Autodesk Inventor part; units mm, degrees
ref_plane "YZ Plane" through (0, 0, 0) normal (1, 0, 0) x (0, 1, 0)
ref_plane "XZ Plane" through (0, 0, 0) normal (0, 1, 0) x (-1, 0, 0)
ref_plane "XY Plane" through (0, 0, 0) normal (0, 0, 1) x (1, 0, 0)
sketch "Sketch1" plane through (0, 0, 0) normal (0, 1, 0) x (-1, 0, 0)
  line L0 (-16.8496, 81.8638) -> (105.0704, 81.8638)
  line L1 (105.0704, 81.8638) -> (105.0704, -7.0362)
  line L2 (105.0704, -7.0362) -> (-16.8496, -7.0362)
  line L3 (-16.8496, -7.0362) -> (-16.8496, 81.8638)
  point P0 (0, 0)
  dimension "d0" = 121.92
  dimension "d1" = 88.9
extrude "Extrusion1" add sketch "Sketch1" along normal blind 3.429
sketch "Sketch2" plane through (0, 3.429, 0) normal (0, 1, 0) x (1, 0, 0)
  line L0 (-105.0704, -81.8638) -> (16.8496, -81.8638)
  line L1 (16.8496, 7.0362) -> (-105.0704, 7.0362)
  line L2 (-105.0704, 7.0362) -> (-105.0704, -81.8638)
  circle A0 centre (-98.7204, -2.6158) radius 1.5875
  circle A1 centre (-98.7204, -72.2118) radius 1.5875
  circle A2 centre (-4.7404, -2.6158) radius 1.5875
  circle A3 centre (-4.7404, -72.2118) radius 1.5875
  point P0 (0, 0)
  dimension "d4" = 121.92
  dimension "d5" = 88.9
  dimension "d6" = 6.35
  dimension "d8" = 6.35
  dimension "d12" = 3.175
  dimension "d13" = 3.175
  dimension "d15" = 3.175
  dimension "d18" = 93.98
  dimension "d20" = 69.596
  dimension "d21" = 9.652
  dimension "d22" = 9.652
  dimension "d23" = 3.175
  dimension "d64" = 9.652
  dimension "d65" = 9.652
extrude "Extrusion3" cut sketch "Sketch2" against normal through all
sketch "Sketch4" plane through (0, 3.429, 0) normal (0, 1, 0) x (1, 0, 0)
  circle A0 centre (-98.7204, -2.6158) radius 1.5875
  circle A1 centre (-98.7204, -72.2118) radius 1.5875
  line L0 (16.8496, 7.0362) -> (-105.0704, 7.0362)
  line L1 (-105.0704, 7.0362) -> (-105.0704, -81.8638)
  line L2 (-101.8954, -78.6888) -> (-47.0314, -78.6888)
  line L3 (-47.0314, -78.6888) -> (-47.0314, 3.8612)
  line L4 (-47.0314, 3.8612) -> (-101.8954, 3.8612)
  line L5 (-101.8954, 3.8612) -> (-101.8954, -78.6888)
  circle A2 centre (-98.7204, -2.6158) radius 3.175
  circle A3 centre (-98.7204, -72.2118) radius 3.175
  point P0 (0, 0)
  dimension "d26" = 54.864
  dimension "d27" = 82.55
  dimension "d28" = 3.175
  dimension "d29" = 3.175
  dimension "d38" = 3.175
extrude "Extrusion4" add sketch "Sketch4" along normal blind 2.54 contours L5 L4 L3 L2
sketch "Sketch5" plane through (0, 3.429, 0) normal (0, 1, 0) x (1, 0, 0)
  line L0 (-47.0314, 3.8612) -> (-47.0314, -78.6888)
  line L1 (-47.0314, -37.4138) -> (-47.0314, -31.0638)
  line L2 (-47.0314, -31.0638) -> (-47.0314, -43.7638)
  line L3 (-47.0314, -43.7638) -> (-41.9514, -43.7638)
  circle A0 centre (-41.9514, -43.7638) radius 5.08
  circle A1 centre (-41.9514, -31.0638) radius 5.08
  point P0 (0, 0)
  dimension "d35" = 6.35
  dimension "d36" = 12.7
  dimension "d37" = 5.08
extrude "Extrusion5" cut sketch "Sketch5" against normal through all
sketch "Sketch6" plane through (0, 3.429, 0) normal (0, 1, 0) x (1, 0, 0)
  line L0 (-47.0314, -31.0638) -> (-47.0314, -43.7638)
  line L1 (-105.0704, 7.0362) -> (-105.0704, -81.8638)
  line L2 (-47.0314, -37.4138) -> (-40.6814, -37.4138)
  line L3 (-40.6814, -37.4138) -> (-40.6814, -65.3538)
  line L4 (-40.6814, -65.3538) -> (-40.6814, 3.1754)
  line L5 (-40.6814, 3.1754) -> (12.6586, 3.1754)
  line L6 (12.6586, 3.1754) -> (12.6586, -65.3538)
  line L7 (12.6586, -65.3538) -> (-40.6814, -65.3538)
  line L8 (-40.6814, -65.3538) -> (-40.6814, -63.0678)
  line L9 (-40.6814, -63.0678) -> (12.6586, -63.0678)
  line L10 (-40.6814, -63.0678) -> (-33.0614, -63.0678)
  line L11 (-33.0614, -63.0678) -> (-5.1214, -63.0678)
  circle A0 centre (-33.0614, -63.0678) radius 3.175
  circle A1 centre (-5.1214, -63.0678) radius 3.175
  line L12 (-40.6814, 3.1754) -> (-38.3954, 3.1754)
  line L13 (-38.3954, 3.1754) -> (-38.3954, -65.3538)
  line L14 (-38.3954, 3.1754) -> (-38.3954, -10.6168)
  circle A2 centre (-38.3954, -10.6168) radius 3.175
  line L15 (10.3726, 3.1754) -> (10.3726, -11.7598)
  circle A3 centre (10.3726, -11.7598) radius 3.175
  point P0 (0, 0)
  dimension "d39" = 6.35
  dimension "d40" = 27.94
  dimension "d41" = 68.5292
  dimension "d42" = 53.34
  dimension "d43" = 2.286
  dimension "d44" = 7.62
  dimension "d45" = 27.94
  dimension "d46" = 6.35
  dimension "d47" = 6.35
  dimension "d48" = 2.286
  dimension "d49" = 13.7922
  dimension "d50" = 6.35
  dimension "d51" = 14.9352
  dimension "d52" = 2.286
  dimension "d53" = 6.35
extrude "Extrusion6" add sketch "Sketch6" along normal blind 3.81 contours A2 L4 | L4 A2 L13 | L13 A2 | A0 L9 | L9 A0 L7 | L7 A0 | A1 L9 | L9 A1 L7 | L7 A1 | A3 L6 | A3 L6
sketch "Sketch7" plane through (-38.3954, 7.239, 10.6168) normal (0, 1, 0) x (1, 0, 0)
  circle A0 centre (48.768, -1.143) radius 3.175
  circle A1 centre (33.274, -52.451) radius 3.175
  circle A2 centre (5.334, -52.451) radius 3.175
  circle A3 centre (48.768, -1.143) radius 1.27
  point P0 (38.3954, 10.6168)
  dimension "d56" = 2.54
extrude "Extrusion7" add sketch "Sketch7" along normal blind 2.54 contours A3
sketch "Sketch8" plane through (-38.3954, 7.239, 10.6168) normal (0, 1, 0) x (1, 0, 0)
  circle A0 centre (0, 0) radius 3.175
  circle A1 centre (5.334, -52.451) radius 3.175
  circle A2 centre (33.274, -52.451) radius 3.175
  circle A3 centre (0, 0) radius 1.0605
  circle A4 centre (5.334, -52.451) radius 1.0605
  circle A5 centre (33.274, -52.451) radius 1.0604
  point P0 (38.3954, 10.6168)
  dimension "d59" = 2.1209
  dimension "d60" = 2.1209
  dimension "d61" = 2.1209
extrude "Extrusion8" cut sketch "Sketch8" against normal through all contours A3 | A4 | A5
properties part number "base_plate_r2"
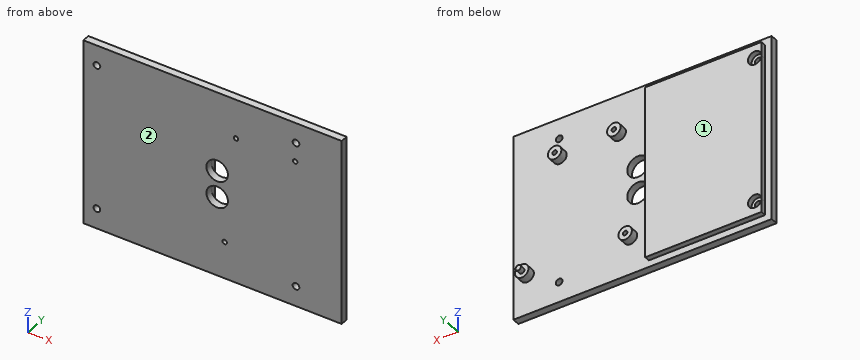
Design review of the part built by this model. Coordinates are the model's own, in mm. Face numbers are marked on the shaded views. A direction names the side the tool comes from. Round coordinates to 2 decimals unless told otherwise and drop trailing zeros. Write each loop counter-clockwise with the first axis right and the second up, starting at its lowest first coordinate (ties: lowest second). Pieces come first, ordered by that corner, then holes. Notation, with made-up numbers: (68, 31) -> (95, 31) arc R15 cw to (95, 54) -> close; hole circle Ø6 at (18, -13.5). An arc over 180 degrees is marked (long way). One line per item, written item: value. Start each with the question number.
Q1. Add section B-B (x = -52). Give the boundary of the cut face in (y, z), then the cut area to 3 significant figures.
Q2. Add section D-D (x = -17). Give the boundary of the cut face in (y, z).
Q3. Add section A-A (z = 47.5). Give the boundary of the cut face in (x, y), then the cut area to 3 significant figures.
Q4. Tool access review of the marked faces 1 and 2: name each direction out of +Z, -Z, +X, -X, +Y, -Y from which nothing blocks a thin tool from reaching the whole face with its end or side.
Q5. To check wall thickness, follow probe 1 along Y at (x, z) = (5, 16.5); probe 2 along Y at (x, z) = (-92.5, 30); probe 3 along X at (y, z) = (4.5, 6). State the ranges of each line that lie inside material, in increasing order.
Q6. Add section C-C (z = 24.5). Give the boundary of the cut face in (x, y), then the cut area to 3 significant figures.
Q7. Insertion check: P1, Ø7, axis at x = -6, z = 63, coming from the +Y side; P2, Ø1.5, axis at x = -12, y = 6, coming from the -Z side (1 decimal); P3, Ø2, axis at y = 5, z = 50, coming from the -X side; P4, Ø2, axis at x = -69, y = 5, coming from the -Z side. Each pin has a flat end and moves straight along its axis. Give the tip position at first contact, or say it passes through.
Response:
1. outline: (0, -7.04) -> (3.43, -7.04) -> (3.43, -3.86) -> (5.97, -3.86) -> (5.97, 78.69) -> (3.43, 78.69) -> (3.43, 81.86) -> (0, 81.86) -> close
1. area: 515 mm^2
2. outline: (0, -7.04) -> (3.43, -7.04) -> (3.43, 81.86) -> (0, 81.86) -> close
3. outline: (-105.07, 0) -> (-45.39, 0) -> (-45.39, 3.43) -> (-47.03, 3.43) -> (-47.03, 5.97) -> (-101.9, 5.97) -> (-101.9, 3.43) -> (-105.07, 3.43) -> close; (-38.51, 0) -> (16.85, 0) -> (16.85, 3.43) -> (-38.51, 3.43) -> close
3. area: 534 mm^2
4. face 1: +Z, -Z, -X, +Y
4. face 2: +Z, -Z, +X, -X, -Y
5. probe 1: y = 0 to 3.43
5. probe 2: y = 0 to 5.97
5. probe 3: x = -101.9 to -47.03
6. outline: (-105.07, 0) -> (16.85, 0) -> (16.85, 3.43) -> (-47.03, 3.43) -> (-47.03, 5.97) -> (-101.9, 5.97) -> (-101.9, 3.43) -> (-105.07, 3.43) -> close
6. area: 557 mm^2
7. P1: stops at y = 7.24
7. P2: passes through
7. P3: stops at x = -101.9
7. P4: stops at z = -3.86
